```python
from build123d import *

# Parameters (mm, degrees)
F0_W     = 38.1
F0_H     = 6.35
F1_DEPTH = 6.35


with BuildPart() as f1:
    # F0 (on Front) → F1 (new body)
    with BuildSketch(Plane.XZ):
        with BuildLine():
            Line((-114.3, -12.7), (114.3, -12.7))
            Line((114.3, -12.7), (114.3, 12.7))
            Line((114.3, 12.7), (107.95, 12.7))
            Line((107.95, 12.7), (107.95, 38.1))
            Line((107.95, 38.1), (114.3, 38.1))
            Line((114.3, 38.1), (114.3, 63.5))
            Line((114.3, 63.5), (107.95, 63.5))
            Line((107.95, 63.5), (107.95, 88.9))
            Line((107.95, 88.9), (114.3, 88.9))
            Line((114.3, 88.9), (114.3, 114.3))
            Line((114.3, 114.3), (50.8, 114.3))
            ThreePointArc((50.8, 114.3), (41.819744, 110.580256), (38.1, 101.6))
            Line((38.1, 101.6), (38.1, 25.4))
            ThreePointArc((38.1, 25.4), (34.380256, 16.419744), (25.4, 12.7))
            Line((25.4, 12.7), (-25.4, 12.7))
            ThreePointArc((-25.4, 12.7), (-34.380256, 16.419744), (-38.1, 25.4))
            Line((-38.1, 25.4), (-38.1, 101.6))
            ThreePointArc((-38.1, 101.6), (-41.819744, 110.580256), (-50.8, 114.3))
            Line((-50.8, 114.3), (-114.3, 114.3))
            Line((-114.3, 114.3), (-114.3, 88.9))
            Line((-114.3, 88.9), (-107.95, 88.9))
            Line((-107.95, 88.9), (-107.95, 63.5))
            Line((-107.95, 63.5), (-114.3, 63.5))
            Line((-114.3, 63.5), (-114.3, 38.1))
            Line((-114.3, 38.1), (-107.95, 38.1))
            Line((-107.95, 38.1), (-107.95, 12.7))
            Line((-107.95, 12.7), (-114.3, 12.7))
            Line((-114.3, 12.7), (-114.3, -12.7))
        make_face()
        with Locations((-63.5, 0)):
            Rectangle(F0_W, F0_H, mode=Mode.SUBTRACT)
        with Locations((63.5, 0)):
            Rectangle(F0_W, F0_H, mode=Mode.SUBTRACT)
    extrude(amount=F1_DEPTH)


solid = f1.part
```
Input: part model. Units: mm. Frame: model coordinates. A direction names the side the tool comes from. Give positions to 0.01 mm unless a question says otherwise; leave off trailing zeros. Order: outer loops, then holes, each group sorted by start corner. A loop starts at its lowest first (then second) coordinate and runs counter-clockwise, first axis right, second up.
1. Pin query (flat end, axial travel): pin 1 Ø1.9 at (y, z) = (-4, 21) entering from +X; pin 2 Ø1.9 at (x, y) = (6, -3) entering from +Z. Return the tip coordinate at first contact, or that it passes through.
Computed:
pin 1: stops at x = 107.95
pin 2: stops at z = 12.7
2. Cut plane D-D (y = -3.25). State how many separate pieces and enclosed holes the cut face has, and give its area (3 significant figures).
Computed:
separate pieces: 1
enclosed holes: 2
area: 20,200 mm2
3. Cut plane C-C (x = 14). Return loops of the section in (y, z).
Computed:
outline: (-6.35, -12.7) - (0, -12.7) - (0, 12.7) - (-6.35, 12.7) - close
4. Cut plane A-A (z = 51). Return loops of the section in (x, y), and give its area (3 significant figures).
Computed:
outline: (-114.3, -6.35) - (-38.1, -6.35) - (-38.1, 0) - (-114.3, 0) - close; (38.1, -6.35) - (114.3, -6.35) - (114.3, 0) - (38.1, 0) - close
area: 968 mm2
5. Cut plane B-B (x = 66.5). Return loops of the section in (y, z) (3 decimals), and give its area (3 significant figures).
Computed:
outline: (-6.35, -12.7) - (0, -12.7) - (0, -3.175) - (-6.35, -3.175) - close; (-6.35, 3.175) - (0, 3.175) - (0, 114.3) - (-6.35, 114.3) - close
area: 766 mm2
6. Draft query along Z for faces 1 (the face through (0, -3, 12.7)), 2 (the face through (-114.3, -3, 0)), 3 (the face through (-82.55, -3, 0)). Return one class per face: released by +Z, released by -Z, zero draft, split by the parting line, or undercut.
Computed:
face 1: released by +Z
face 2: zero draft
face 3: undercut
7. Line query: probe 1 along X at (y, z) = (-2.75, -2.5); probe 2 along Z at (x, y) = (-69.5, -3.75) (3 decimals); probe 3 along X at (y, z) = (-6, 64.5). Output: solid intervals per line, ascending.
Computed:
probe 1: x = -114.3 to -82.55, -44.45 to 44.45, 82.55 to 114.3
probe 2: z = -12.7 to -3.175, 3.175 to 114.3
probe 3: x = -107.95 to -38.1, 38.1 to 107.95
8. Set-up query: faces 4 (the face through (-107.95, -3, 76)), 5 (the face through (-34.28, -3.13, 16.32)), 6 (the face through (-2, -3, -12.7)), 7 (the face through (-64, -3, -3.175)). Return all of +Z, -Z, +X, -X, +Y, -Y with unobstructed straight access to the full face (end or side cutting, diameter ignored); none if empty.
Computed:
face 4: -X, +Y, -Y
face 5: +Z, +Y, -Y
face 6: -Z, +X, -X, +Y, -Y
face 7: +Y, -Y
